```python
from build123d import *

# Parameters (mm, degrees)
PAD_DEPTH       = 58
POCKET_DEPTH    = 10
SKETCH002_R     = 11
POCKET001_DEPTH = 4
SKETCH003_R     = 14.5
SKETCH003_R_2   = 11
PAD001_DEPTH    = 3
SKETCH004_R     = 11
POCKET002_DEPTH = 4
SKETCH005_R     = 14.5
SKETCH005_R_2   = 11
PAD002_DEPTH    = 3
SKETCH006_R     = 3.15
POCKET003_DEPTH = 10
SKETCH007_R     = 7.5
POCKET004_DEPTH = 199.001
CHAMFER_SIZE    = 2.99


with BuildPart() as part:
    # Sketch → Pad (new body)
    with BuildSketch(Plane.XZ):
        with BuildLine():
            Line((0, 125), (0, 0))
            Line((0, 0), (196, 0))
            Line((196, 0), (196, 125))
            Line((196, 125), (186, 125))
            Line((186, 125), (186, 25))
            ThreePointArc((171, 10), (181.606602, 14.393398), (186, 25))
            Line((171, 10), (25, 10))
            ThreePointArc((10, 25), (14.393398, 14.393398), (25, 10))
            Line((10, 25), (10, 125))
            Line((10, 125), (0, 125))
        make_face()
    extrude(amount=PAD_DEPTH)

    # Sketch001 (on DatumPlane) → Pocket (cut)
    with BuildSketch(Plane.YZ.offset(196)):
        with BuildLine():
            Line((-40, 47.7), (-40, 44.7))
            ThreePointArc((-40, 44.7), (-29, 33.7), (-18, 44.7))
            Line((-18, 47.7), (-18, 44.7))
            Line((-18, 47.7), (-18, 50.7))
            ThreePointArc((-18, 50.7), (-29, 61.7), (-40, 50.7))
            Line((-40, 47.7), (-40, 50.7))
        make_face()
        with BuildLine():
            Line((-42.75, 60.2), (-42.75, 63.2))
            Line((-42.75, 63.2), (-42.75, 66.2))
            ThreePointArc((-42.75, 66.2), (-44.5, 67.95), (-46.25, 66.2))
            Line((-46.25, 66.2), (-46.25, 63.2))
            Line((-46.25, 63.2), (-46.25, 60.2))
            ThreePointArc((-46.25, 60.2), (-44.5, 58.45), (-42.75, 60.2))
        make_face()
        with BuildLine():
            Line((-11.75, 63.2), (-11.75, 60.2))
            ThreePointArc((-15.25, 60.2), (-13.5, 58.45), (-11.75, 60.2))
            Line((-15.25, 63.2), (-15.25, 60.2))
            Line((-15.25, 66.2), (-15.25, 63.2))
            ThreePointArc((-11.75, 66.2), (-13.5, 67.95), (-15.25, 66.2))
            Line((-11.75, 63.2), (-11.75, 66.2))
        make_face()
        with BuildLine():
            Line((-46.25, 35.2), (-46.25, 32.2))
            Line((-46.25, 29.200012), (-46.25, 32.2))
            ThreePointArc((-46.25, 29.200012), (-44.500006, 27.450012), (-42.75, 29.2))
            Line((-42.75, 32.2), (-42.75, 29.2))
            Line((-42.75, 35.2), (-42.75, 32.2))
            ThreePointArc((-42.75, 35.2), (-44.5, 36.95), (-46.25, 35.2))
        make_face()
        with BuildLine():
            Line((-11.75, 35.2), (-11.75, 32.2))
            Line((-11.75, 32.2), (-11.75, 29.2))
            ThreePointArc((-15.25, 29.2), (-13.5, 27.45), (-11.75, 29.2))
            Line((-15.25, 29.2), (-15.25, 32.2))
            Line((-15.25, 32.2), (-15.25, 35.2))
            ThreePointArc((-11.75, 35.2), (-13.5, 36.95), (-15.25, 35.2))
        make_face()
    extrude(amount=-POCKET_DEPTH, mode=Mode.SUBTRACT)

    # Sketch002 (on DatumPlane) → Pocket001 (cut)
    with BuildSketch(Plane.YZ.offset(196)):
        with Locations((-29, 96)):
            Circle(SKETCH002_R)
    extrude(amount=-POCKET001_DEPTH, mode=Mode.SUBTRACT)

    # Sketch003 (on DatumPlane) → Pad001 (join)
    with BuildSketch(Plane.YZ.offset(196)):
        with Locations((-29, 96)):
            Circle(SKETCH003_R)
        with Locations((-29, 96)):
            Circle(SKETCH003_R_2, mode=Mode.SUBTRACT)
    extrude(amount=PAD001_DEPTH)

    # Sketch004 → Pocket002 (cut)
    with BuildSketch(Plane.YZ):
        with Locations((-29, 96)):
            Circle(SKETCH004_R)
    extrude(amount=POCKET002_DEPTH, mode=Mode.SUBTRACT)

    # Sketch005 → Pad002 (join)
    with BuildSketch(Plane.YZ):
        with Locations((-29, 96)):
            Circle(SKETCH005_R)
        with Locations((-29, 96)):
            Circle(SKETCH005_R_2, mode=Mode.SUBTRACT)
    extrude(amount=-PAD002_DEPTH)

    # Sketch006 → Pocket003 (cut)
    with BuildSketch(Plane.XY):
        with Locations((98, -29)):
            Circle(SKETCH006_R)
    extrude(amount=POCKET003_DEPTH, mode=Mode.SUBTRACT)

    # Sketch007 (on DatumPlane) → Pocket004 (cut, through all)
    with BuildSketch(Plane.YZ.offset(196)):
        with Locations((-29, 96)):
            Circle(SKETCH007_R)
        with BuildLine():
            ThreePointArc((0, 96), (-29, 125), (-58, 96))
            Line((-58, 96), (-68, 96))
            Line((-68, 96), (-68, 136))
            Line((-68, 136), (10, 136))
            Line((10, 136), (10, 96))
            Line((10, 96), (0, 96))
        make_face()
    extrude(amount=-POCKET004_DEPTH, mode=Mode.SUBTRACT)

    # Chamfer
    chamfer_edges = [part.edges().sort_by_distance(p)[0] for p in [
        (0, -43.5, 96),
        (196, -43.5, 96),
    ]]
    chamfer(chamfer_edges, length=CHAMFER_SIZE)


solid = part.part
```
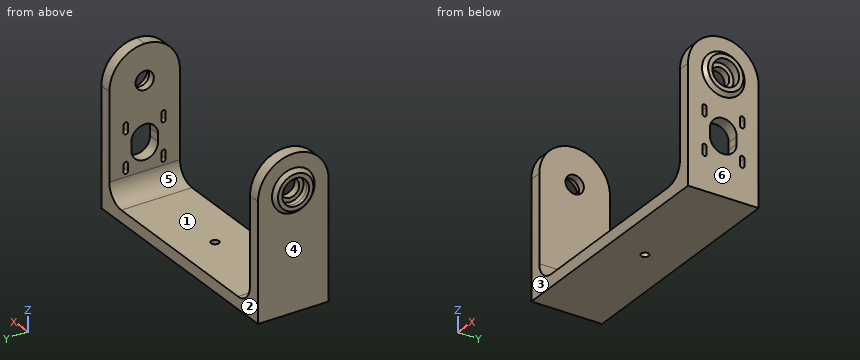
Check sheet for the modelled part. Datum: model origin and axes. Units: mm. Face numbers are marked on the shaded views. A direction names the side the tool comes from. Coordinates: 2 decimals unless noted, no trailing zeros. Write each loop counter-clockwise with the first axis right and the second up, starting at its lowest first coordinate (ties: lowest second). Pieces come first, ordered by that corner, then holes. Notation, with made-up numbers: (71.5, 36.25) -> (99.5, 36.25) arc R17 ccw to (99.5, 59.25) -> close; hole circle Ø11 at (1.25, 32). An arc over 180 degrees is marked (long way). Use a Markdown table: item, result.
1. Sectioned sample at C-C (y = -54). Enter the section's corners in (x, z), plus the area to 3 significant figures.
Reported:
| item | result |
|---|---|
| outline | (0, 0) -> (196, 0) -> (196, 110.7) -> (186, 110.7) -> (186, 25) arc R15 cw to (171, 10) -> (25, 10) arc R15 cw to (10, 25) -> (10, 110.7) -> (0, 110.7) -> close |
| area | 4,070 mm2 |
2. Sectioned sample at A-A (z = 75). Enter the section's corners in (x, y).
Reported:
| item | result |
|---|---|
| outline | (0, -58) -> (10, -58) -> (10, 0) -> (0, 0) -> close; (186, -58) -> (196, -58) -> (196, 0) -> (186, 0) -> close |
3. Scan lines: line 1 along Z through (x, y) = (188.8, -29); line 2 along Z through (x, y) = (6, -29); line 3 along X through (y, z) = (-10, 35). Record each from-to range of solid material in increasing order.
Reported:
| item | result |
|---|---|
| line 1 | z = 0 to 33.7, 61.7 to 88.5, 103.5 to 125 |
| line 2 | z = 0 to 88.5, 103.5 to 125 |
| line 3 | x = 0 to 10, 186 to 196 |
4. Release check for a two-part mould opening along X. For the marked faces 3, 4, 5 and 6 record: pulls with the +X half, pulls with the -X half, needs draft (parallel to the pull), parting line crosses it, or undercut.
Reported:
| item | result |
|---|---|
| face 3 | needs draft |
| face 4 | pulls with the -X half |
| face 5 | undercut |
| face 6 | pulls with the +X half |
5. Sectioned sample at B-B (x = 98). Enter the section's corners in (y, z).
Reported:
| item | result |
|---|---|
| outline | (-58, 0) -> (-32.15, 0) -> (-32.15, 10) -> (-58, 10) -> close; (-25.85, 0) -> (0, 0) -> (0, 10) -> (-25.85, 10) -> close |
6. Sectioned sample at D-D (x = 155). Enter the section's corners in (y, z), plus the area to 3 significant figures.
Reported:
| item | result |
|---|---|
| outline | (-58, 0) -> (0, 0) -> (0, 10) -> (-58, 10) -> close |
| area | 580 mm2 |
7. Go/stop test with flat-tipped pins: pin 1 Ø17 at (y, z) = (-29, 96) entering from +X; pin 2 Ø3 at (x, z) = (189, 31.5) entering from +Y; pin 3 Ø8 at (y, z) = (-8, 30) entering from -X; pin 4 Ø10 at (y, z) = (-50.5, 110.5) entering from +X. Record where each tip stops, or that it passes through.
Reported:
| item | result |
|---|---|
| pin 1 | stops at x = 192 |
| pin 2 | stops at y = 0 |
| pin 3 | stops at x = 0 |
| pin 4 | stops at x = 196 |
8. Tool access check on the marked faces 1 and 2. Record the directions out of +Z, -Z, +X, -X, +Y, -Y that give a thin tool (end or side, any length) a straight path to the whole face; none if there is none.
Reported:
| item | result |
|---|---|
| face 1 | +Z, +Y, -Y |
| face 2 | +Z, -Z, +X, -X, +Y |
